Autodesk Inventor part; units mm, degrees
ref_plane "YZ Plane" through (0, 0, 0) normal (1, 0, 0) x (0, 1, 0)
ref_plane "XZ Plane" through (0, 0, 0) normal (0, 1, 0) x (-1, 0, 0)
ref_plane "XY Plane" through (0, 0, 0) normal (0, 0, 1) x (1, 0, 0)
sketch "Sketch1" plane through (0, 0, 0) normal (0, 1, 0) x (-1, 0, 0)
  line L0 (7.1393, -6.0921) -> (-0.2013, -6.0921)
  line L1 (-0.2013, -6.0921) -> (-3.8716, 0.2651)
  line L2 (-3.8716, 0.2651) -> (-0.2013, 6.6222)
  line L3 (-0.2013, 6.6222) -> (7.1393, 6.6222)
  line L4 (7.1393, -6.0921) -> (10.8096, 0.2651)
  line L5 (10.8096, 0.2651) -> (7.1393, 6.6222)
  point P0 (0, 0)
  dimension "d0" = 7.3406
  dimension "d1" = 7.3406
  dimension "d2" = 7.3406
  dimension "d3" = 7.3406
  dimension "d4" = 120
  dimension "d5" = 120
  dimension "d6" = 120
  dimension "d7" = 7.3406
  dimension "d8" = 120
  dimension "d9" = 7.3406
extrude "Extrusion1" add sketch "Sketch1" along normal blind 254
sketch "Sketch3" plane through (0, 254, 0) normal (0, 1, 0) x (1, 0, 0)
  circle A0 centre (-3.469, -0.2651) radius 4.699
  point P0 (0, 0)
  dimension "d21" = 9.398
extrude "Extrusion2" add sketch "Sketch3" along normal blind 7.112
chamfer "Chamfer1" distance 0.5 angle 45 1 edges at (-8.168, 261.112, 0.2651)
sketch "Sketch4" plane through (-3.469, 261.112, 0.2651) normal (0, 1, 0) x (1, 0, 0)
  circle A0 centre (0, 0) radius 4.199
  circle A1 centre (0, 0) radius 3.1877
  point P0 (3.469, 0.2651)
  dimension "d27" = 6.3754
extrude "Extrusion3" add sketch "Sketch4" along normal blind 12.7 contours A1
chamfer "Chamfer2" distance 0.5 angle 45 1 edges at (-6.6567, 273.812, 0.2651)
sketch "Sketch5" plane through (0, 0, 0) normal (0, -1, 0) x (1, 0, 0)
  line L0 (-7.1393, -6.0921) -> (0.2013, -6.0921)
  line L1 (0.2013, -6.0921) -> (3.8716, 0.2651)
  line L2 (3.8716, 0.2651) -> (0.2013, 6.6222)
  line L3 (0.2013, 6.6222) -> (-7.1393, 6.6222)
  line L4 (-7.1393, 6.6222) -> (-10.8096, 0.2651)
  line L5 (-10.8096, 0.2651) -> (-7.1393, -6.0921)
  point P0 (0, 0)
extrude "Extrusion4" cut sketch "Sketch5" against normal blind 101.346
sketch "Sketch6" plane through (0, 101.346, 0) normal (0, -1, 0) x (1, 0, 0)
  line L0 (0.2013, -6.0921) -> (-7.1393, -6.0921)
  line L1 (3.8716, 0.2651) -> (0.2013, -6.0921)
  line L2 (0.2013, 6.6222) -> (3.8716, 0.2651)
  line L3 (-7.1393, 6.6222) -> (0.2013, 6.6222)
  line L4 (-10.8096, 0.2651) -> (-7.1393, 6.6222)
  line L5 (-7.1393, -6.0921) -> (-10.8096, 0.2651)
  point P0 (0, 0)
extrude "Extrusion5" add sketch "Sketch6" along normal blind 7.3406
sketch "Sketch7" plane through (0, 94.0054, 0) normal (0, -1, 0) x (1, 0, 0)
  circle A0 centre (-3.469, 0.2651) radius 2.4892
  point P0 (0, 0)
  dimension "d37" = 4.9784
extrude "Extrusion6" cut sketch "Sketch7" against normal blind 15.875
sketch "Sketch8" plane through (-3.469, 109.8804, 0.2651) normal (0, -1, 0) x (1, 0, 0)
  circle A0 centre (0, 0) radius 2.4892
  point P0 (3.469, -0.2651)
fillet "Fillet1" radius 1.3462 1 edges at (-5.9582, 109.8804, 0.2651)
equation "\"d5\" = d4"
equation "\"d8\" = d4"
properties part number "Hex Shaft"
Build history of the part. All positions in model axes, mm. A direction names the side the tool comes from. Give positions to 0.01 mm unless a question says otherwise; leave off trailing zeros. Loops run counter-clockwise (first coordinate to the right, second up) from the corner with the lowest first, then second, coordinate; pieces in that order, holes last.
Item 1: Drill centre lines: line 1 (Y direction, x = -3.5, z = -5.25); line 2 (Y direction, x = -2.75, z = 0.75); line 3 (X direction, y = 227, z = 6.25). Where is each one in solid material? Low to high.
Answers follow:
line 1: y = 94.01 to 254
line 2: y = 109.88 to 273.81
line 3: x = -7.35 to 0.42
Item 2: Which spindle directions (+Z, -Z, +X, -X, +Y, -Y) get a long thin tool onto all of the face, cutting with end or side? Do faces 5 (the face through (-7, 261.112, -1)), 6 (the face through (2.06, 175.12, -2.87)). Say none if no direction does.
Answers follow:
face 5: +Y
face 6: -Z, +X, +Y, -Y
Item 3: Slice it at A-A, the plane y = 189. List the corners of the cut face in (x, z).
Answers follow:
outline: (-10.81, 0.27) - (-7.14, -6.09) - (0.2, -6.09) - (3.87, 0.27) - (0.2, 6.62) - (-7.14, 6.62) - close
Item 4: Pull direction X, two halves, no side cores. Call faces 1 (the face through (-4, 175, 6.622)), 2 (the face through (2.01, 175.12, 3.49)), 3 (the face through (-5.444, 101.168, -1.25)), 4 (the face through (-5.82, 267.13, 2.42)): released by +X, released by -X, zero draft, split by the parting line, or undercut.
Answers follow:
face 1: zero draft
face 2: released by +X
face 3: undercut
face 4: split by the parting line
Item 5: Flat gauge pin, fed straight in: pin 1 (1.1 mm diameter, centred on x = -3.5, z = 0.5, fed in from -Y). Where does the tip first touch, or does it go through?
Answers follow:
pin 1: stops at y = 109.88
